from build123d import *

# Parameters (mm, degrees)
SKETCH_1_W          = 59
SKETCH_1_H          = 85
SKETCH_1_W_2        = 41
SKETCH_1_H_2        = 21
EXTRUDE_1_DEPTH     = 4
SKETCH_2_R          = 1.6
SKETCH_2_W          = 6.65
SKETCH_2_H          = 1.3
CUT_EXTRUDE_1_DEPTH = 4
SKETCH_5_R          = 3
CUT_EXTRUDE_4_DEPTH = 10
SKETCH_3_R          = 3
CUT_EXTRUDE_2_DEPTH = 4
FILLET_1_R          = 25
FILLET_2_R          = 3
SKETCH_4_R          = 1.6
CUT_EXTRUDE_3_DEPTH = 10
EXTRUDE_2_DEPTH     = 4
FILLET_3_R          = 1
FILLET_4_R          = 5
SKETCH_8_R          = 1.6
CUT_EXTRUDE_5_DEPTH = 10


with BuildPart() as part:
    # ｽｹｯﾁ1 → ﾎﾞｽ - 押し出し1 (new body)
    with BuildSketch(Plane.XY):
        with Locations((2.5, 11.5)):
            Rectangle(SKETCH_1_W, SKETCH_1_H)
        with Locations((0, 25.5)):
            Rectangle(SKETCH_1_W_2, SKETCH_1_H_2, mode=Mode.SUBTRACT)
    extrude(amount=EXTRUDE_1_DEPTH)

    # ｽｹｯﾁ2 → ｶｯﾄ - 押し出し1 (cut)
    with BuildSketch(Plane(origin=(0, 0, 0), x_dir=(-1, 0, 0), z_dir=(0, 0, -1))):
        with Locations((-24.3, 20.55)):
            Circle(SKETCH_2_R)
        with Locations((-24.3, 30.45)):
            Circle(SKETCH_2_R)
        with Locations((24.3, 30.45)):
            Circle(SKETCH_2_R)
        with Locations((24.3, 20.55)):
            Circle(SKETCH_2_R)
        with Locations((-23.825, 25.5)):
            Rectangle(SKETCH_2_W, SKETCH_2_H)
        with Locations((23.825, 25.5)):
            Rectangle(SKETCH_2_W, SKETCH_2_H)
    extrude(amount=-CUT_EXTRUDE_1_DEPTH, mode=Mode.SUBTRACT)

    # ｽｹｯﾁ5 → ｶｯﾄ - 押し出し4 (cut)
    with BuildSketch(Plane.XY.offset(4)):
        with Locations((-10.2, -2.5)):
            Circle(SKETCH_5_R)
    extrude(amount=-CUT_EXTRUDE_4_DEPTH, mode=Mode.SUBTRACT)

    # ｽｹｯﾁ3 → ｶｯﾄ - 押し出し2 (cut)
    with BuildSketch(Plane.XY.offset(4)):
        with Locations((-10.2, 42.5)):
            Circle(SKETCH_3_R)
        with Locations((-10.2, -19.5)):
            Circle(SKETCH_3_R)
    extrude(amount=-CUT_EXTRUDE_2_DEPTH, mode=Mode.SUBTRACT)

    # ﾌｨﾚｯﾄ1
    fillet_1_edges = [part.edges().sort_by_distance(p)[0] for p in [
        (-27, 54, 2),
        (-27, -31, 2),
    ]]
    fillet(fillet_1_edges, radius=FILLET_1_R)

    # ﾌｨﾚｯﾄ2
    fillet_2_edges = [part.edges().sort_by_distance(p)[0] for p in [
        (32, 54, 2),
        (32, -31, 2),
    ]]
    fillet(fillet_2_edges, radius=FILLET_2_R)

    # ｽｹｯﾁ4 → ｶｯﾄ - 押し出し3 (cut)
    with BuildSketch(Plane.XY.offset(4)):
        with Locations((27, 49)):
            Circle(SKETCH_4_R)
        with Locations((27, -26)):
            Circle(SKETCH_4_R)
    extrude(amount=-CUT_EXTRUDE_3_DEPTH, mode=Mode.SUBTRACT)

    # ｽｹｯﾁ6 → ﾎﾞｽ - 押し出し2 (add)
    with BuildSketch(Plane.XY.offset(4)):
        Polygon((-27, 19.5), (-43.945270358, 19.5), (-38.364198183, 11.5), (-43.945270358, 3.5), (-27, 3.5), align=None)
    extrude(amount=-EXTRUDE_2_DEPTH)

    # ﾌｨﾚｯﾄ3
    fillet_3_edges = [part.edges().sort_by_distance(p)[0] for p in [
        (-38.364198183, 11.5, 2),
    ]]
    fillet(fillet_3_edges, radius=FILLET_3_R)

    # ﾌｨﾚｯﾄ4
    fillet_4_edges = [part.edges().sort_by_distance(p)[0] for p in [
        (-27, 19.5, 2),
        (-27, 3.5, 2),
    ]]
    fillet(fillet_4_edges, radius=FILLET_4_R)

    # ｽｹｯﾁ8 → ｶｯﾄ - 押し出し5 (cut)
    with BuildSketch(Plane.XY.offset(4)):
        with Locations((2, -26)):
            Circle(SKETCH_8_R)
        with Locations((2, 49)):
            Circle(SKETCH_8_R)
    extrude(amount=-CUT_EXTRUDE_5_DEPTH, mode=Mode.SUBTRACT)


solid = part.part
Read the model definition and answer for the solid it produces. Units are mm, in the model's axes. A direction names the side the tool comes from. Coordinates: 2 decimals unless noted, no trailing zeros. Order: outer loops, then holes, each group sorted by start corner. A loop starts at its lowest first (then second) coordinate and runs counter-clockwise, first axis right, second up. Notation, with made-up numbers: M -37,36 L -17,36 A28 cw -17,62 Z; hole C 13.5,68.5 d9. An arc over 180 degrees is marked long. Put each result on its own line as item: value. Start each with the question number.
Item 1: Section D-D, the plane x = -24.3 is taken. Determine the outline of the cut face in (y, z).
Item 2: Given pin 1 Ø2.5 at (x, y) = (27, -26) entering from +Z; pin 2 Ø1.2 at (x, z) = (-22.5, 1.5) entering from +Y; pin 3 Ø2 at (y, z) = (-13, 1) entering from -X; pin 4 Ø2 at (y, z) = (42, 1) entering from -X, each flat-ended and moving along its own axis, determine where each tip first touches the part or whether it passes through.
Item 3: For faces 4 (the face through (-20.5, 31, 2)), 5 (the face through (-27, -4, 2)), 6 (the face through (-41.318, 7.266, 2.028)), determine the directions among +Z, -Z, +X, -X, +Y, -Y from which every point of the face is accessible in a straight line to the end or side of a thin tool.
Item 4: Consider probe 1 along Y at (x, z) = (27, 1); probe 2 along Y at (x, z) = (23, 3.75); probe 3 along Y at (x, z) = (-10, 2.65). Determine where each line is inside the solid, lowest interval first. Write a range as [from, to].
Item 5: Section C-C, the plane x = -10.2 is taken. Determine the outline of the cut face in (y, z).
Item 6: The mould has two halves that part along X. Classify faces 1 (the face through (20.5, 31, 2)), 2 (the face through (2, 12, 0)), 3 (the face through (31.14, 53.1, 2.03)): +X half, -X half, draft (parallel to the pull), parting line (faces both ways), or undercut.
Item 7: Section A-A, the plane y = -26 is taken. Determine the outline of the cut face in (x, z), plus the area to 3 significant figures.
Item 8: Section B-B, the plane y = -2.5 is taken. Determine the outline of the cut face in (x, z).
Computed:
1. outline: M -17.3,0 L 18.95,0 L 18.95,4 L -17.3,4 Z; M 22.15,0 L 24.85,0 L 24.85,4 L 22.15,4 Z; M 26.15,0 L 28.85,0 L 28.85,4 L 26.15,4 Z; M 32.05,0 L 40.3,0 L 40.3,4 L 32.05,4 Z
2. pin 1: passes through
2. pin 2: stops at y = 44.13
2. pin 3: stops at x = -26.27
2. pin 4: stops at x = -23.93
3. face 4: +Z, -Z
3. face 5: +Z, -Z, -X, -Y
3. face 6: +Z, -Z, -X
4. probe 1: y = [-31, -27.6], [-24.4, 24.85], [26.15, 47.4], [50.6, 54]
4. probe 2: y = [-31, 19.62], [21.48, 24.85], [26.15, 29.52], [31.38, 54]
4. probe 3: y = [-29.69, -22.49], [-16.51, -5.49], [0.49, 15], [36, 39.51], [45.49, 52.69]
5. outline: M -29.62,0 L -22.5,0 L -22.5,4 L -29.62,4 Z; M -16.5,0 L -5.5,0 L -5.5,4 L -16.5,4 Z; M 0.5,0 L 15,0 L 15,4 L 0.5,4 Z; M 36,0 L 39.5,0 L 39.5,4 L 36,4 Z; M 45.5,0 L 52.62,0 L 52.62,4 L 45.5,4 Z
6. face 1: undercut
6. face 2: draft
6. face 3: +X half
7. outline: M -17,0 L 0.4,0 L 0.4,4 L -17,4 Z; M 3.6,0 L 25.4,0 L 25.4,4 L 3.6,4 Z; M 28.6,0 L 32,0 L 32,4 L 28.6,4 Z
7. area: 170 mm2
8. outline: M -27,0 L -13.2,0 L -13.2,4 L -27,4 Z; M -7.2,0 L 32,0 L 32,4 L -7.2,4 Z
